Work out the finished part from the listing and answer in its coordinate system (mm). A direction names the side the tool comes from. Give positions to 0.01 mm unless a question says otherwise; leave off trailing zeros. Loops run counter-clockwise (first coordinate to the right, second up) from the corner with the lowest first, then second, coordinate; pieces in that order, holes last. Notation, with made-up numbers: (40, 78) - (87, 78) arc R20 ccw to (87, 117) - close; hole circle Ø10 at (71.25, -5). An arc over 180 degrees is marked (long way). Use CSV: the item, a comma, the result in double quotes.
from build123d import *

# Parameters (mm, degrees)
EXTRUDE_1_DEPTH     = 8
SKETCH_2_R          = 2
CUT_EXTRUDE_1_DEPTH = 6
SKETCH_3_R          = 2
EXTRUDE_2_DEPTH     = 6


with BuildPart() as part:
    # 草图1 → 凸台-拉伸1 (new body)
    with BuildSketch(Plane.XY):
        Polygon((0, 3), (-2.598076211, 1.5), (-2.598076211, -1.5), (0, -3), (2.598076211, -1.5), (2.598076211, 1.5), align=None)
    extrude(amount=EXTRUDE_1_DEPTH)

    # 草图2 → 切除-拉伸1 (cut)
    with BuildSketch(Plane.XY.offset(8)):
        Circle(SKETCH_2_R)
    extrude(amount=-CUT_EXTRUDE_1_DEPTH, mode=Mode.SUBTRACT)

    # 草图3 → 凸台-拉伸2 (add)
    with BuildSketch(Plane(origin=(0, 0, 0), x_dir=(-1, 0, 0), z_dir=(0, 0, -1))):
        with Locations(Location((0, 0, 0), (0, 0, 180))):
            Circle(SKETCH_3_R)
    extrude(amount=EXTRUDE_2_DEPTH)


solid = part.part
Item 1: A cutting plane is placed at D-D on z = -5. Determine the outline of the cut face in (x, y), and give its area (3 significant figures).
Determined:
outline,"circle Ø4 at (0, 0)"
area,"12.6 mm²"
Item 2: A cutting plane is placed at B-B on y = 0. Determine the outline of the cut face in (x, z).
Determined:
outline,"(-2.6, 0) - (-2, 0) - (-2, -6) - (2, -6) - (2, 0) - (2.6, 0) - (2.6, 8) - (2, 8) - (2, 2) - (-2, 2) - (-2, 8) - (-2.6, 8) - close"
Item 3: The mould has two halves that part along Y. Classify faces 1 (the flat face through (2.598, 0, 4)), 2 (the flat face through (0, 0, 2)), 3 (the flat face through (-1.28, 2.26, 3.94)): pulls with the +Y half, pulls with the -Y half, needs draft (parallel to the pull), parting line crosses it, or undercut.
Determined:
face 1,"needs draft"
face 2,"undercut"
face 3,"pulls with the +Y half"
Item 4: A cutting plane is placed at C-C on x = -0.75. Determine the outline of the cut face in (y, z), and give its area (3 significant figures).
Determined:
outline,"(-2.57, 0) - (-1.85, 0) - (-1.85, -6) - (1.85, -6) - (1.85, 0) - (2.57, 0) - (2.57, 8) - (1.85, 8) - (1.85, 2) - (-1.85, 2) - (-1.85, 8) - (-2.57, 8) - close"
area,"41.1 mm²"
Item 5: For faces 4 (the cylindrical face through (0, -2, 5)), 5 (the cylindrical face through (0, 2, -3)), 6 (the flat face through (-1.32, -2.24, 3.94)), determine the directions among +Z, -Z, +X, -X, +Y, -Y from which every point of the face is accessible in a straight line to the end or side of a thin tool.
Determined:
face 4,"+Z"
face 5,"-Z"
face 6,"+Z, -Z, -X, -Y"
Item 6: A cutting plane is placed at A-A on z = 4.25. Determine the outline of the cut face in (x, y).
Determined:
outline,"(-2.6, -1.5) - (0, -3) - (2.6, -1.5) - (2.6, 1.5) - (0, 3) - (-2.6, 1.5) - close; hole circle Ø4 at (0, 0)"
Item 7: Find the intervals of material crossed by line 1 (Z direction, x = -0.6, y = 2.45); line 2 (Z direction, x = -1.2, y = -0.35); line 3 (Y direction, x = 0.1, z = 6.75), in increasing order.
Determined:
line 1,"z = 0 to 8"
line 2,"z = -6 to 2"
line 3,"y = -2.94 to -2, 2 to 2.94"
Item 8: Given P1, Ø1, axis at x = 1, z = -3, coming from the -Y side; P2, Ø3, axis at x = 0, y = 0, coming from the +Z side, each flat-ended and moving along its own axis, determine where each tip first touches the part or whether it passes through.
Determined:
P1,"stops at y = -1.94"
P2,"stops at z = 2"
